Study the drawing (mm; zero at the part's minimum x, y, z) and answer. Give positions to 0.01 mm unless a question says otherwise; leave off trailing zeros. Loops run counter-clockwise (first coordinate to the right, second up) from the corner with the lowest first, then second, coordinate; pieces in that order, holes last. Notation, with made-up numbers: (35.25, 12.25) - (78.25, 12.25) arc R16 ccw to (78.25, 35.25) - close; hole circle Ø9 at (37, 85). An arc over 180 degrees is marked (long way). One line per item, written item: value. Start each with the question number.
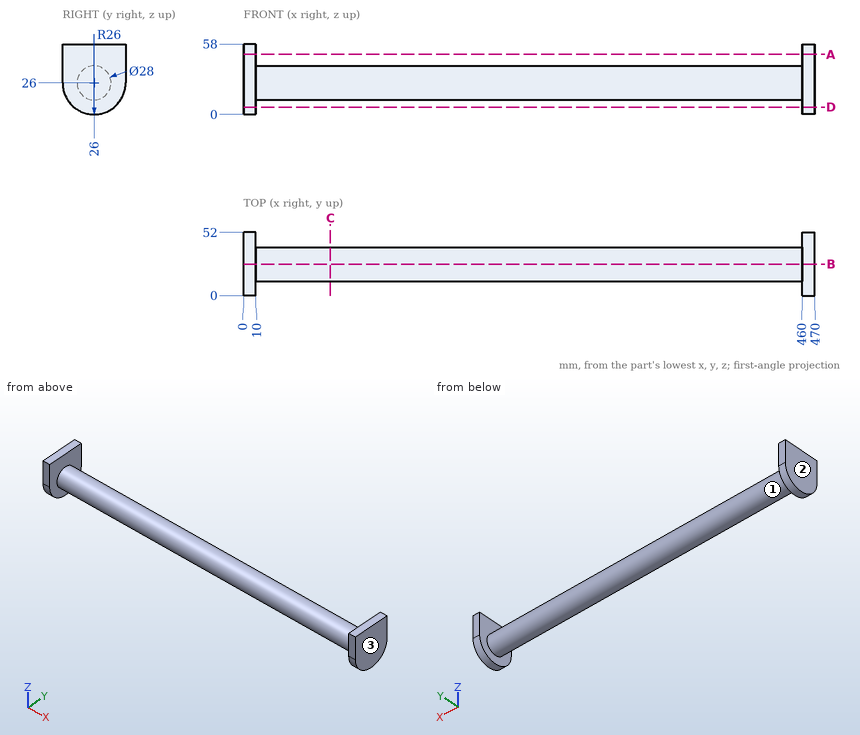
1. Flat-ended cylindrical pins translate along their axes: pin 1 (10 mm diameter, centred on x = 413, y = 12.5, fed in from +Z); pin 2 (12 mm diameter, centred on x = 288.5, z = 50, fed in from +Y); pin 3 (8 mm diameter, centred on x = 220.5, z = 34.5, fed in from -Y); pin 4 (1.5 mm diameter, centred on x = 123.5, z = 19.5, fed in from +Y). Find the tip coordinate at first contact, or state that the pin passes through.
2. A cutting plane is placed at C-C (x = 71.5). Determine the outline of the cut face in (y, z).
3. Find the intervals of material crossed by L1, parallel to X at y = 21, z = 48; L2, parallel to Z at x = 200.5, y = 26; L3, parallel to Z at x = 417, y = 28, in increasing order. Write a range as [from, to].
4. A cutting plane is placed at B-B (y = 26). Determine the outline of the cut face in (x, z), plus the area to 3 significant figures.
5. Determine the mould class of the marked faces 1, 2 and 3 for opening direction X: released by +X, released by -X, zero draft, split by the parting line, or undercut.
6. A cutting plane is placed at D-D (z = 6). Determine the outline of the cut face in (x, y), plus the area to 3 significant figures.
7. A cutting plane is placed at A-A (z = 49.5). Determine the outline of the cut face in (x, y).
Results below:
1. pin 1: stops at z = 37.12
1. pin 2: passes through
1. pin 3: stops at y = 12.74
1. pin 4: stops at y = 38.76
2. outline: circle Ø28 at (26, 26)
3. L1: x = [0, 10], [460, 470]
3. L2: z = [12, 40]
3. L3: z = [12.14, 39.86]
4. outline: (0, 0) - (10, 0) - (10, 12) - (460, 12) - (460, 0) - (470, 0) - (470, 58) - (460, 58) - (460, 40) - (10, 40) - (10, 58) - (0, 58) - close
4. area: 13,800 mm^2
5. face 1: undercut
5. face 2: released by -X
5. face 3: released by +X
6. outline: (0, 9.39) - (10, 9.39) - (10, 42.61) - (0, 42.61) - close; (460, 9.39) - (470, 9.39) - (470, 42.61) - (460, 42.61) - close
6. area: 665 mm^2
7. outline: (0, 0) - (10, 0) - (10, 52) - (0, 52) - close; (460, 0) - (470, 0) - (470, 52) - (460, 52) - close
